Here's the drawing with two shaded views (mm, measured from the low corner). I have some questions. A direction names the side the tool comes from. Coordinates: 2 decimals unless noted, no trailing zeros. Order: outer loops, then holes, each group sorted by start corner. A loop starts at its lowest first (then second) coordinate and runs counter-clockwise, first axis right, second up. Notation, with made-up numbers: (4.5, -14.5) -> (53.5, -14.5) arc R13 cw to (53.5, -6.5) -> close; hole circle Ø3 at (-11.5, 28.5). An arc over 180 degrees is marked (long way). Answer in a Markdown table with one row per item. Add a question column.
1. We'd pull the mould along X, two halves only. Please class the marked faces 1, 2 and 3: pulls with the +X half, pulls with the -X half, needs draft (parallel to the pull), parting line crosses it, or undercut.
2. Imagine slicing it at C-C on y = 18.25. Write out the boundary of the cut face in (x, z).
3. Will this pin go through, and if not, where does the flat tip stop? pin 1 (3 mm diameter, centred on x = 42.5, z = 81, fed in from +Y).
4. Imagine slicing it at D-D on z = 18.5. Write out the boundary of the cut face in (x, y), plus the area to 3 significant figures.
5. On a 3-axis mill with a long thin cutter (end or side, diameter ignored), from which of +Z, -Z, +X, -X, +Y, -Y can I reach the whole of each face in a straight line? I mean the marked faces 4 and 5. Say none if no direction works.
6. Imagine slicing it at B-B on x = 110. Write out the boundary of the cut face in (y, z).
7. If I drill on line 1 along Z through (x, y) = (110, 12.25); line 2 along X through (y, z) = (10, 110); line 3 along X through (y, z) = (3.75, 102), over which ranges is the centre line in solid material (lowest first)? Write a range as [from, to].
8. Imagine slicing it at A-A on z = 110. Write out the boundary of the cut face in (x, y), plus the area to 3 significant figures.
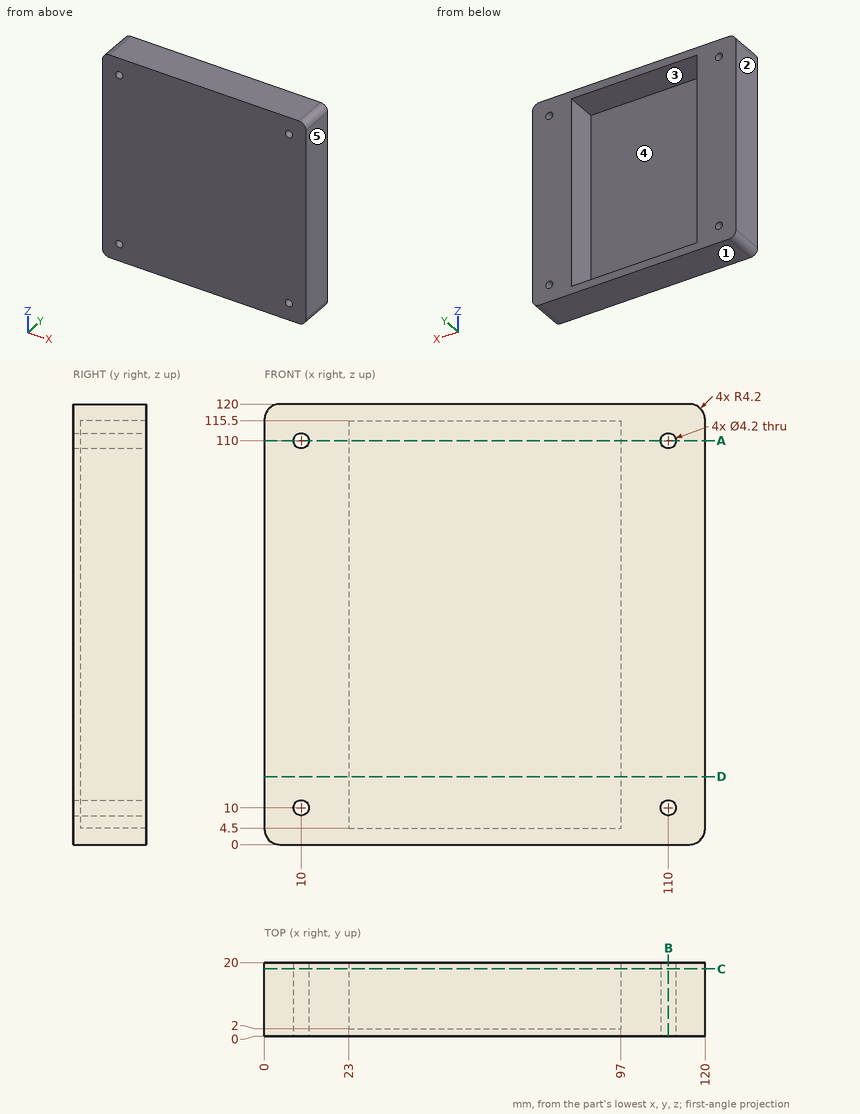
Answers follow:
| question | item | result |
|---|---|---|
| 1 | face 1 | needs draft |
| 1 | face 2 | pulls with the -X half |
| 1 | face 3 | undercut |
| 2 | outline | (0, 4.2) arc R4.2 ccw to (4.2, 0) -> (115.8, 0) arc R4.2 ccw to (120, 4.2) -> (120, 115.8) arc R4.2 ccw to (115.8, 120) -> (4.2, 120) arc R4.2 ccw to (0, 115.8) -> close; hole circle Ø4.2 at (10, 10); hole circle Ø4.2 at (10, 110); hole (23, 4.5) -> (97, 4.5) -> (97, 115.5) -> (23, 115.5) -> close; hole circle Ø4.2 at (110, 10); hole circle Ø4.2 at (110, 110) |
| 3 | pin 1 | stops at y = 2 |
| 4 | outline | (0, 0) -> (120, 0) -> (120, 20) -> (97, 20) -> (97, 2) -> (23, 2) -> (23, 20) -> (0, 20) -> close |
| 4 | area | 1,070 mm² |
| 5 | face 4 | +Y |
| 5 | face 5 | +Z, -Z, +X, +Y, -Y |
| 6 | outline | (0, 0) -> (20, 0) -> (20, 7.9) -> (0, 7.9) -> close; (0, 12.1) -> (20, 12.1) -> (20, 107.9) -> (0, 107.9) -> close; (0, 112.1) -> (20, 112.1) -> (20, 120) -> (0, 120) -> close |
| 7 | line 1 | z = [0, 7.9], [12.1, 107.9], [112.1, 120] |
| 7 | line 2 | x = [0, 7.9], [12.1, 23], [97, 107.9], [112.1, 120] |
| 7 | line 3 | x = [0, 23], [97, 120] |
| 8 | outline | (0, 0) -> (7.9, 0) -> (7.9, 20) -> (0, 20) -> close; (12.1, 0) -> (107.9, 0) -> (107.9, 20) -> (97, 20) -> (97, 2) -> (23, 2) -> (23, 20) -> (12.1, 20) -> close; (112.1, 0) -> (120, 0) -> (120, 20) -> (112.1, 20) -> close |
| 8 | area | 900 mm² |
